from build123d import *

# Parameters (mm, degrees)
F1_DEPTH = 150
F3_T     = -5
F4_R     = 50
F5_DEPTH = 5


with BuildPart() as f1:
    # F0 (on Top) → F1 (new body)
    with BuildSketch(Plane.XY):
        with BuildLine():
            Line((0, 640), (0, 0))
            Line((0, 0), (360, 0))
            Line((360, 0), (360, 490))
            ThreePointArc((360, 490), (316.066017, 596.066017), (210, 640))
            Line((210, 640), (0, 640))
        make_face()
    extrude(amount=F1_DEPTH)

    # F2: F1 across plane


with BuildPart() as f1_1:
    add(f1.part)
    add(f1.part.mirror(Plane.XY))

    # F3
    f3_openings = [f1_1.faces().sort_by_distance(p)[0] for p in [
        (180, 0, 0),
    ]]
    offset(amount=F3_T, openings=f3_openings)

    # F4 (on face) → F5 (cut, through all)
    with BuildSketch(Plane(origin=(0, 0, 0), x_dir=(0, -1, 0), z_dir=(-1, 0, 0))):
        with Locations((-100, 0)):
            Circle(F4_R)
    extrude(amount=-F5_DEPTH, mode=Mode.SUBTRACT)


solid = f1_1.part
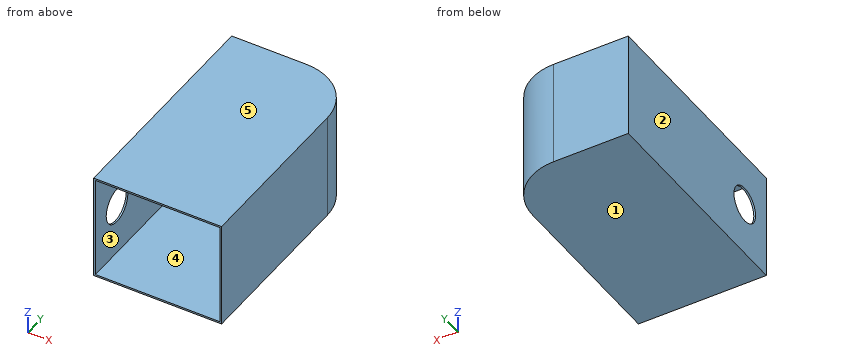
Can you work these out from the model? Positions are in its coordinate system, mm. Face numbers are marked on the shaded views. A direction names the side the tool comes from. Coordinates: 2 decimals unless noted, no trailing zeros. Write each loop counter-clockwise with the first axis right and the second up, starting at its lowest first coordinate (ties: lowest second). Pieces come first, ordered by that corner, then holes. Notation, with made-up numbers: (-25.75, 51.25) -> (5.25, 51.25) arc R5 ccw to (5.25, 59.25) -> close; hole circle Ø6 at (85.5, 62.5). An arc over 180 degrees is marked (long way). Write each question's results on one line, items separated by ' | '. Start each with the question number.
Q1. Imagine slicing it at B-B (y = 394.5). Write out the boundary of the cut face in (x, z), then the cut area to 3 significant figures.
Q2. Imagine slicing it at D-D (y = 100). Write out the boundary of the cut face in (x, z).
Q3. Imagine slicing it at C-C (z = 111.5). Write out the boundary of the cut face in (x, y), then the cut area to 3 significant figures.
Q4. We'd pull the mould along X, two halves only. Please class the marked faces 1, 2 and 3: +X half, -X half, draft (parallel to the pull), parting line (faces both ways), or undercut.
Q5. On a 3-axis mill with a long thin cutter (end or side, diameter ignored), from which of +Z, -Z, +X, -X, +Y, -Y can I reach the whole of each face in a straight line? I mean the marked faces 4 and 5. Say none if no direction works.
Q6. Imagine slicing it at A-A (z = 0). Write out the boundary of the cut face in (x, y), then the cut area to 3 significant figures.
Q7. I'm going to push flat-ended pins straight in: pin 1 (8 mm diameter, centred on x = 85.5, z = -69.5, fed in from -Y); pin 2 (2 mm diameter, centred on y = 103.5, z = -27, fed in from -X); pin 3 (1.5 mm diameter, centred on x = 306.5, z = -81, fed in from +Y). Where does each tip first touch, or does it pass through?
Q8. If I drill on probe 1 along Z at (x, y) = (68, 245); probe 2 along X at (y, z) = (383, -46.5); probe 3 along Z at (x, y) = (1.5, 100), over which ranges is the centre line in solid material (lowest first)?
Taken from the geometry:
1) outline: (0, -150) -> (360, -150) -> (360, 150) -> (0, 150) -> close; hole (5, -145) -> (355, -145) -> (355, 145) -> (5, 145) -> close | area: 6,500 mm^2
2) outline: (0, -150) -> (360, -150) -> (360, 150) -> (0, 150) -> (0, 50) -> (5, 50) -> (5, 145) -> (355, 145) -> (355, -145) -> (5, -145) -> (5, -50) -> (0, -50) -> close
3) outline: (0, 0) -> (5, 0) -> (5, 635) -> (210, 635) arc R145 cw to (355, 490) -> (355, 0) -> (360, 0) -> (360, 490) arc R150 ccw to (210, 640) -> (0, 640) -> close | area: 7,830 mm^2
4) face 1: draft | face 2: -X half | face 3: undercut
5) face 4: -Y | face 5: +Z, +X, -X, +Y, -Y
6) outline: (0, 0) -> (5, 0) -> (5, 50) -> (0, 50) -> close; (0, 150) -> (5, 150) -> (5, 635) -> (210, 635) arc R145 cw to (355, 490) -> (355, 0) -> (360, 0) -> (360, 490) arc R150 ccw to (210, 640) -> (0, 640) -> close | area: 7,330 mm^2
7) pin 1: stops at y = 635 | pin 2: stops at x = 355 | pin 3: stops at y = 605.46
8) probe 1: z = -150 to -145, 145 to 150 | probe 2: x = 0 to 5, 355 to 360 | probe 3: z = -150 to -50, 50 to 150
